from build123d import *

# Parameters (mm, degrees)
F0_W     = 16.2
F0_H     = 1.2
F1_DEPTH = 4.5
F2_W     = 16.2
F2_H     = 0.675
F2_H_2   = 1.2
F2_H_3   = 3.125
F3_DEPTH = 0.8
F5_E28_W = 22.0063713977
F5_E28_H = 4.5
F5_E29_W = 12.0937982574
F5_E29_H = 4.5
F5_E30_W = 12.0937982574
F5_E30_H = 4.5
F5_E31_W = 11.5652361646
F5_E31_H = 4.5
F5_E32_W = 11.5652361646
F5_E32_H = 4.5
F6_DEPTH = 0.4


with BuildPart() as f1:
    # F0 (on Top) → F1 (new body)
    with BuildSketch(Plane.XY):
        with Locations((-29.7626322135, 18.7695161968)):
            Rectangle(F0_W, F0_H)
    extrude(amount=F1_DEPTH)



with BuildPart() as f1b:
    # F0 (on Top) → F1, piece 2 (new body)
    with BuildSketch(Plane.XY):
        with Locations((-29.7626322135, 16.2195161968)):
            Rectangle(F0_W, F0_H)
    extrude(amount=F1_DEPTH)


with BuildPart() as f1_1:
    add(f1.part)

    add(f1b.part)  # F3 merges F1b
    # F2 (on face) → F3 (join)
    with BuildSketch(Plane.XY.offset(4.5)):
        Polygon((-47.8626322135, 41.1793105304), (-37.8626322135, 17.4945161968), (-21.6626322135, 17.4945161968), (-21.6626322135, 22.4945161968), (-21.6626322135, 33.4945161968), (-47.8626322135, 45.7203537226), align=None)
        Polygon((-21.6626322135, 22.4945161968), (-21.6626322135, 17.4945161968), (-21.6626322135, 16.8195161968), (-21.6626322135, 15.6195161968), (-21.6626322135, 12.4945161968), (-6.3626514748, 12.4945161968), (-6.3626514748, 22.4945161968), align=None)
        with Locations((-29.7626322135, 17.1570161968)):
            Rectangle(F2_W, F2_H)
        with Locations((-29.7626322135, 16.2195161968)):
            Rectangle(F2_W, F2_H_2)
        with Locations((-29.7626322135, 14.0570161968)):
            Rectangle(F2_W, F2_H_3)
    extrude(amount=F3_DEPTH)

    # F5_E28 (on explicit) + F5_E29 (on explicit) + F5_E30 (on explicit) + F5_E31 (on explicit) + F5_E32 (on explicit) → F6 (join, symmetric)
    with BuildSketch(Plane(origin=(-47.8626322135, 43.4498321265, 4.5), x_dir=(0.9061941294, -0.4228619158, 0), z_dir=(0.4228619158, 0.9061941294, 0))):
        with Locations((11.0031856988, 2.25)):
            Rectangle(F5_E28_W, F5_E28_H)
    with BuildSketch(Plane(origin=(-18.4564497322, 19.9771542102, 4.5), x_dir=(1, 0, 0), z_dir=(0, 1, 0))):
        with Locations((6.0468991287, 2.25)):
            Rectangle(F5_E29_W, F5_E29_H)
    with BuildSketch(Plane(origin=(-18.4564497322, 14.4476536661, 4.5), x_dir=(1, 0, 0), z_dir=(0, 1, 0))):
        with Locations((6.0468991287, 2.25)):
            Rectangle(F5_E30_W, F5_E30_H)
    with BuildSketch(Plane(origin=(-21.6626322135, 31.073756516, 4.5), x_dir=(-1, 0, 0), z_dir=(0, -1, 0))):
        with Locations((5.7826180823, 2.25)):
            Rectangle(F5_E31_W, F5_E31_H)
    with BuildSketch(Plane(origin=(-21.6626322135, 26.7479624599, 4.5), x_dir=(-1, 0, 0), z_dir=(0, -1, 0))):
        with Locations((5.7826180823, 2.25)):
            Rectangle(F5_E32_W, F5_E32_H)
    extrude(amount=F6_DEPTH, both=True, dir=(0.4228619158, 0.9061941294, 0))


solid = f1_1.part
Can you work these out from the model? Positions are in its coordinate system, mm. A direction names the side the tool comes from. Coordinates: 2 decimals unless noted, no trailing zeros. Loops run counter-clockwise (first coordinate to the right, second up) from the corner with the lowest first, then second, coordinate; pieces in that order, holes last. Notation, with made-up numbers: M -16,76.5 L -3,76.5 A26 ccw -3,108.5 Z; hole C 7,14 d4. An arc over 180 degrees is marked long. Answer as CSV lines item,"result". Start each with the question number.
1. Thinking about a two-plate mould opening in Y: for faces 1 (the face through (-21.663, 16, 2)), 2 (the face through (-28, 30.711, 2)), 3 (the face through (-12, 20.34, 2)), 4 (the face through (-32, 26, 4.5)), which applies, +Y half, -Y half, draft (parallel to the pull), parting line (faces both ways), or undercut?
2. Suppose I cut it at B-B, the plane x = -36.5. List the corners of the cut face in (y, z) for me.
3. For pin 1 Ø1.5 at (y, z) = (39.5, 1.5) entering from +X; pin 2 Ø1 at (y, z) = (19, 2) entering from -X; pin 3 Ø1.3 at (x, z) = (-14, 1.5) entering from +Y, each with a flat end and sliding along its axis, tell me the tip position at first contact or that it passes through.
4. Suppose I cut it at D-D, the plane x = -25. List the corners of the cut face in (y, z) for me.
5. Suppose I cut it at C-C, the plane y = 35. List the corners of the cut face in (x, z) for me, plus the area to 3 significant figures.
6. For faces 5 (the face through (-38.2, 38.5, 2.2)), 6 (the face through (-37.862, 39.225, 2.218)), 7 (the face through (-30, 19.37, 2)), which set-ups out of +Z, -Z, +X, -X, +Y, -Y let a thin tool reach every point of the face, with its end or its side?
7. If I drill on probe 1 along Y at (x, z) = (-27, 3.7); probe 2 along Y at (x, z) = (-29, 1.15); probe 3 along Y at (x, z) = (-30.5, 0.7), over which ranges is the centre line in solid material (lowest first)? Write a range as [from, to].
8. Suppose I cut it at A-A, the plane z = 2.4. List the corners of the cut face in (x, y) for me, plus the area to 3 significant figures.
Output:
1,face 1,"draft"
1,face 2,"undercut"
1,face 3,"+Y half"
1,face 4,"undercut"
2,outline,"M 12.49,4.5 L 15.62,4.5 L 15.62,0 L 16.82,0 L 16.82,4.5 L 18.17,4.5 L 18.17,0 L 19.37,0 L 19.37,4.5 L 37.71,4.5 L 37.71,0 L 38.59,0 L 38.59,4.5 L 40.42,4.5 L 40.42,5.3 L 12.49,5.3 Z"
3,pin 1,"stops at x = -36.84"
3,pin 2,"stops at x = -37.86"
3,pin 3,"stops at y = 20.34"
4,outline,"M 12.49,4.5 L 15.62,4.5 L 15.62,0 L 16.82,0 L 16.82,4.5 L 18.17,4.5 L 18.17,0 L 19.37,0 L 19.37,4.5 L 26.39,4.5 L 26.39,0 L 27.11,0 L 27.11,4.5 L 30.71,4.5 L 30.71,0 L 31.44,0 L 31.44,4.5 L 35.05,4.5 L 35.05,5.3 L 12.49,5.3 Z"
5,outline,"M -45.25,4.5 L -30.7,4.5 L -30.7,0 L -28.81,0 L -28.81,4.5 L -24.89,4.5 L -24.89,5.3 L -45.25,5.3 Z"
5,area,"24.8 mm^2"
6,face 5,"-Z, -X"
6,face 6,"-Z, +X, +Y"
6,face 7,"-Z, +X, -X"
7,probe 1,"y = [15.62, 16.82], [18.17, 19.37], [26.39, 27.11], [30.71, 31.44]"
7,probe 2,"y = [15.62, 16.82], [18.17, 19.37], [26.39, 27.11], [30.71, 31.44], [34.21, 35.09]"
7,probe 3,"y = [15.62, 16.82], [18.17, 19.37], [26.39, 27.11], [30.71, 31.44], [34.91, 35.79]"
8,outline,"M -48.03,43.09 L -28.09,33.78 L -27.75,34.51 L -47.69,43.81 Z; M -37.86,15.62 L -21.66,15.62 L -21.66,16.82 L -37.86,16.82 Z; M -37.86,18.17 L -21.66,18.17 L -21.66,19.37 L -37.86,19.37 Z; M -33.4,26.39 L -21.83,26.39 L -21.49,27.11 L -33.06,27.11 Z; M -33.4,30.71 L -21.83,30.71 L -21.49,31.44 L -33.06,31.44 Z; M -18.63,14.09 L -6.53,14.09 L -6.19,14.81 L -18.29,14.81 Z; M -18.63,19.61 L -6.53,19.61 L -6.19,20.34 L -18.29,20.34 Z"
8,area,"90.8 mm^2"
